Read the model definition and answer for the solid it produces. Units are mm, in the model's axes. A direction names the side the tool comes from. Coordinates: 2 decimals unless noted, no trailing zeros. Order: outer loops, then holes, each group sorted by start corner. A loop starts at its lowest first (then second) coordinate and runs counter-clockwise, first axis right, second up. Notation, with made-up numbers: (71.5, 79.5) -> (109.5, 79.5) arc R29 cw to (109.5, 109.5) -> close; hole circle Ø4 at (55, 82.5). An arc over 180 degrees is marked (long way). Return JSON: item names as keys, results as strings. Group by question number.
```python
from build123d import *

# Parameters (mm, degrees)
SKETCH1_W                     = 101.835629046
SKETCH1_H                     = 3
BOSS_EXTRUDE1_DEPTH           = 12.5
SKETCH2_W                     = 42.486551299
SKETCH2_H                     = 1.8
BOSS_EXTRUDE2_DEPTH           = 45.4
SKETCH3_W                     = 42.486551299
SKETCH3_H                     = 42.486551299
BOSS_EXTRUDE3_DEPTH           = 5
CBORE_FOR_M3_SHCS2_AT_2_COUNT = 2
CBORE_FOR_M3_SHCS2_AT_2_PITCH = 31
CBORE_FOR_M3_SHCS2_AT_3_COUNT = 2
CBORE_FOR_M3_SHCS2_AT_3_PITCH = 43.840620434
CBORE_FOR_M3_SHCS2_AT_4_COUNT = 2
CBORE_FOR_M3_SHCS2_AT_4_PITCH = 31
SKETCH9_R                     = 14.462
CUT_EXTRUDE1_DEPTH            = 10
SKETCH10_W                    = 59.349077747
SKETCH10_H                    = 12.6
BOSS_EXTRUDE4_DEPTH           = 5
SKETCH11_R                    = 2.5
CUT_EXTRUDE2_DEPTH            = 10


with BuildPart() as part:
    # Sketch1 → Boss-Extrude1 (new, symmetric)
    with BuildSketch(Plane(origin=(0, 0, 0), x_dir=(0, 0, -1), z_dir=(1, 0, 0))):
        with Locations((5.332185477, -1.5)):
            Rectangle(SKETCH1_W, SKETCH1_H)
    extrude(amount=BOSS_EXTRUDE1_DEPTH, both=True)

    # Sketch2 → Boss-Extrude2 (add)
    with BuildSketch(Plane.ZY.offset(12.5)):
        with Locations((-35.006724351, -2.1)):
            Rectangle(SKETCH2_W, SKETCH2_H)
    extrude(amount=BOSS_EXTRUDE2_DEPTH)

    # Sketch3 → Boss-Extrude3 (add)
    with BuildSketch(Plane.ZY.offset(12.5)):
        with Locations((-35.006724351, 20.043275649)):
            Rectangle(SKETCH3_W, SKETCH3_H)
    extrude(amount=BOSS_EXTRUDE3_DEPTH)

    # Sketch8 → CBORE for M3 SHCS2 (revolve, cut)
    with BuildSketch(Plane(origin=(-12.5, 4.5, -19.5), x_dir=(0, 0, -1), z_dir=(0, 1, 0))):
        Polygon((0, 0), (0, 45.4), (1.7, 45.4), (1.7, 3), (3.25, 3), (3.25, 0.025), (3.275, 0), align=None)
    cbore_for_m3_shcs2 = revolve(axis=Axis((-6.15, 4.5, -19.5), (-1, 0, 0)), mode=Mode.SUBTRACT)

    # CBORE for M3 SHCS2 at 2: CBORE for M3 SHCS2 ×2
    with Locations(*[(0, 0, -i * CBORE_FOR_M3_SHCS2_AT_2_PITCH) for i in range(1, CBORE_FOR_M3_SHCS2_AT_2_COUNT)]):
        add(cbore_for_m3_shcs2, mode=Mode.SUBTRACT)

    # CBORE for M3 SHCS2 at 3: CBORE for M3 SHCS2 ×2
    with Locations(*[Vector(0, 0.7071067811865476, -0.7071067811865475) * (i * CBORE_FOR_M3_SHCS2_AT_3_PITCH) for i in range(1, CBORE_FOR_M3_SHCS2_AT_3_COUNT)]):
        add(cbore_for_m3_shcs2, mode=Mode.SUBTRACT)

    # CBORE for M3 SHCS2 at 4: CBORE for M3 SHCS2 ×2
    with Locations(*[(0, i * CBORE_FOR_M3_SHCS2_AT_4_PITCH, 0) for i in range(1, CBORE_FOR_M3_SHCS2_AT_4_COUNT)]):
        add(cbore_for_m3_shcs2, mode=Mode.SUBTRACT)

    # Sketch9 → Cut-Extrude1 (cut)
    with BuildSketch(Plane(origin=(-12.5, 0, 0), x_dir=(0, 0, -1), z_dir=(1, 0, 0))):
        with Locations((35, 20)):
            Circle(SKETCH9_R)
    extrude(amount=-CUT_EXTRUDE1_DEPTH, mode=Mode.SUBTRACT)

    # Sketch10 → Boss-Extrude4 (add)
    with BuildSketch(Plane.ZY.offset(12.5)):
        with Locations((15.911090172, 3.3)):
            Rectangle(SKETCH10_W, SKETCH10_H)
    extrude(amount=BOSS_EXTRUDE4_DEPTH)

    # Sketch11 → Cut-Extrude2 (cut)
    with BuildSketch(Plane.ZY.offset(17.5)):
        with Locations((5.95, 5)):
            Circle(SKETCH11_R)
        with Locations((40.574170501, 5)):
            Circle(SKETCH11_R)
    extrude(amount=-CUT_EXTRUDE2_DEPTH, mode=Mode.SUBTRACT)


solid = part.part
```
1. Find section A-A on z = -35. Determine the outline of the cut face in (x, y), and give its area (3 significant figures).
2. Given pin 1 (6 mm diameter, centred on y = 14, z = 8, fed in from +X); pin 2 (6 mm diameter, centred on y = 9.5, z = 9.5, fed in from +X); pin 3 (5.5 mm diameter, centred on x = -16, y = 22, fed in from +Z); pin 4 (4 mm diameter, centred on y = 4.5, z = -19.5, fed in from -X), each flat-ended and moving along its own axis, determine where each tip first touches the part or whether it passes through.
3. Find section C-C on z = 5.95. Determine the outline of the cut face in (x, y), and give its area (3 significant figures).
4. Straight lines are drawn through the part: L1, parallel to Y at x = -16.75, z = -19.5; L2, parallel to X at y = 7, z = 17; L3, parallel to Y at x = -5, z = 10. For each, find the intervals that lie inside material, in ascending order.
5. Which of the six approach directions +Z, -Z, +X, -X, +Y, -Y give full straight-line access (tool end or side, diameter ignored) to faces 1 (the face through (-15.04, 5.75, 42.96)), 2 (the face through (-12.5, 15, -21)), 3 (the face through (-15, 25, -13.763)), 4 (the face through (-14, -3, -17)), 5 (the face through (-15.5, 37, -49))?
6. Find section B-B on y = 20. Determine the outline of the cut face in (x, z), and give its area (3 significant figures).
7. Find section D-D on x = -22. Determine the outline of the cut face in (y, z).
8. For a pull along Z with two mould halves and no side action, classify faces 6 (the face through (-13.992, 4.357, -16.253)), 7 (the face through (-5.8, -0.5, 45.586)), 8 (the face through (-37, -1.2, -35)), 9 (the face through (-13.992, 38.673, -18.795)) as released by +Z, released by -Z, zero draft, split by the parting line, or undercut.
Result:
{
 "1": {"outline": "(-57.9, -3) -> (12.5, -3) -> (12.5, 0) -> (-12.5, 0) -> (-12.5, 5.54) -> (-17.5, 5.54) -> (-17.5, -1.2) -> (-57.9, -1.2) -> close; (-17.5, 34.46) -> (-12.5, 34.46) -> (-12.5, 41.29) -> (-17.5, 41.29) -> close", "area": "225 mm^2"},
 "2": {"pin 1": "through", "pin 2": "x = -12.5", "pin 3": "z = -13.76", "pin 4": "x = -17.5"},
 "3": {"outline": "(-17.5, -3) -> (12.5, -3) -> (12.5, 0) -> (-12.5, 0) -> (-12.5, 2.5) -> (-17.5, 2.5) -> close; (-17.5, 7.5) -> (-12.5, 7.5) -> (-12.5, 9.6) -> (-17.5, 9.6) -> close", "area": "113 mm^2"},
 "4": {"L1": "-3 to 2.8, 6.2 to 33.8, 37.2 to 41.29", "L2": "-17.5 to -12.5", "L3": "-3 to 0"},
 "5": {"face 1": "+X, -X", "face 2": "+Z, -Z, +X, +Y", "face 3": "+Z, +X, -X, +Y", "face 4": "+Z, -Z, +X, -X, -Y", "face 5": "+X"},
 "6": {"outline": "(-17.5, -56.25) -> (-12.5, -56.25) -> (-12.5, -49.46) -> (-17.5, -49.46) -> close; (-17.5, -20.54) -> (-12.5, -20.54) -> (-12.5, -13.76) -> (-17.5, -13.76) -> close", "area": "67.8 mm^2"},
 "7": {"outline": "(-3, -56.25) -> (-1.2, -56.25) -> (-1.2, -13.76) -> (-3, -13.76) -> close"},
 "8": {"face 6": "undercut", "face 7": "released by +Z", "face 8": "zero draft", "face 9": "undercut"}
}
